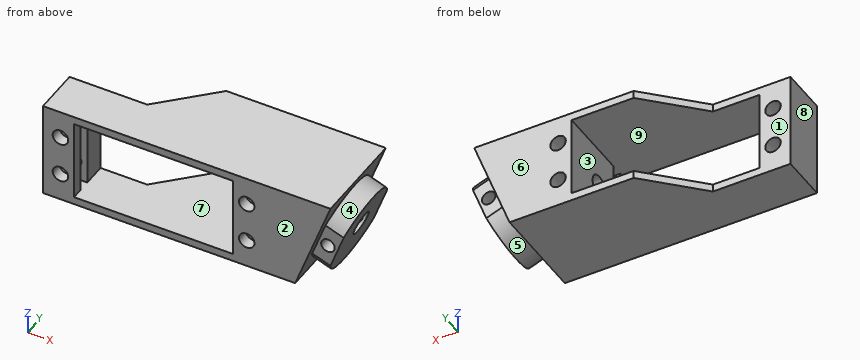
Autodesk Inventor part; units mm, degrees
ref_plane "YZ Plane" through (0, 0, 0) normal (1, 0, 0) x (0, 1, 0)
ref_plane "XZ Plane" through (0, 0, 0) normal (0, 1, 0) x (-1, 0, 0)
ref_plane "XY Plane" through (0, 0, 0) normal (0, 0, 1) x (1, 0, 0)
sketch "Esquisse1" plane through (0, 0, 0) normal (0, 1, 0) x (-1, 0, 0)
  line L0 (20.5, 10.5) -> (-20.5, 10.5)
  line L1 (-20.5, 10.5) -> (-20.5, -10.5)
  line L2 (-20.5, -10.5) -> (20.5, -10.5)
  line L3 (20.5, -10.5) -> (20.5, 10.5)
  line L4 (28.5, 12.5) -> (-36.5, 12.5)
  line L5 (-36.5, 12.5) -> (-36.5, -12.5)
  line L6 (-36.5, -12.5) -> (28.5, -12.5)
  line L7 (28.5, -12.5) -> (28.5, 12.5)
  line L8 (-36.5, -12.5) -> (-45.5993, 12.5)
  line L9 (-45.5993, 12.5) -> (-36.5, 12.5)
  point P0 (0, 0)
  dimension "d0" = 20
  dimension "d1" = 41
  dimension "d2" = 21
  dimension "d3" = 10.5
  dimension "d4" = 20.5
  dimension "d5" = 8
  dimension "d6" = 2
  dimension "d7" = 2
  dimension "d8" = 16
extrude "Extrusion1" add sketch "Esquisse1" along normal mid plane 25
sketch "Esquisse2" plane through (36.5, -12.5, -12.5) normal (0.9397, 0, -0.342) x (-0.342, 0, -0.9397)
  line L0 (-26.6044, 25) -> (0, 0)
  line L1 (0, 0) -> (0, 25)
  line L2 (0, 25) -> (-26.6044, 0)
  arc A0 (-8.3022, 22.298) -> (-18.3022, 22.298) centre (-13.3022, 12.5) ccw
  line L3 (-18.3022, 22.298) -> (-8.3022, 22.298)
  line L4 (-8.3022, 22.298) -> (-8.3022, 2.702)
  line L5 (-8.3022, 2.702) -> (-18.3022, 2.702)
  line L6 (-18.3022, 2.702) -> (-18.3022, 22.298)
  arc A1 (-8.3022, 2.702) -> (-8.3022, 22.298) centre (-13.3022, 12.5) ccw
  arc A2 (-18.3022, 2.702) -> (-8.3022, 2.702) centre (-13.3022, 12.5) ccw
  arc A3 (-18.3022, 22.298) -> (-18.3022, 2.702) centre (-13.3022, 12.5) ccw
  point P0 (0.7376, 12.5)
  dimension "d11" = 22
  dimension "d13" = 10
extrude "Extrusion2" add sketch "Esquisse2" along normal blind 5 contours A3 L6 L0 | L0 L6 L2 A3 | L6 L3 L4 L2 L0 | L0 L2 L6 | L2 L6 A3 | L2 L4 L0 | L0 L4 L5 L6 L2 | A1 L2 L4 | L4 L2 A1 L0 | L0 A1 L4
sketch "Esquisse3" plane through (39.3395, -9.798, -4.6985) normal (0, -1, 0) x (0.9397, 0, -0.342)
  line L0 (5, 10) -> (0, 0)
  line L1 (0, 10) -> (5, 0)
  circle A0 centre (2.5, 5) radius 1.75
  point P0 (-38.574, -9.0398)
  dimension "d16" = 3.5
extrude "Extrusion3" cut sketch "Esquisse3" against normal through all
sketch "Esquisse4" plane through (20.5, -12.5, 10.5) normal (-1, 0, 0) x (0, 0, 1)
  line L0 (-21, 3) -> (0, 3)
  line L1 (0, 3) -> (0, 6)
  line L2 (0, 6) -> (-21, 6)
  line L3 (-21, 6) -> (-21, 3)
  line L4 (-21, 0) -> (-21, 25)
  line L5 (0, 0) -> (0, 25)
  line L6 (0, 0) -> (-21, 0)
  point P0 (-10.5, 12.5)
  dimension "d19" = 3
  dimension "d20" = 3
extrude "Extrusion4" cut sketch "Esquisse4" against normal blind 7 contours L3 L2 L1 L0
sketch "Esquisse5" plane through (-20.5, -12.5, -10.5) normal (1, 0, 0) x (0, 0, -1)
  line L0 (-21, 6) -> (0, 6)
  line L1 (0, 6) -> (0, 3)
  line L2 (0, 3) -> (-21, 3)
  line L3 (-21, 3) -> (-21, 6)
  line L4 (-21, 25) -> (-21, 0)
  line L5 (0, 0) -> (0, 25)
  line L6 (0, 0) -> (-21, 0)
  point P0 (-10.5, 12.5)
  dimension "d23" = 3
  dimension "d24" = 3
extrude "Extrusion5" cut sketch "Esquisse5" against normal blind 7 contours L0 L1 L2 L3
sketch "Esquisse6" plane through (20.5, 12.5, -10.5) normal (-1, 0, 0) x (0, 0, 1)
  line L0 (21, -25) -> (0, 0)
  line L1 (0, -25) -> (21, 0)
  circle A0 centre (10.5, -12.5) radius 3
  dimension "d27" = 6
extrude "Extrusion6" cut sketch "Esquisse6" against normal through all
sketch "Esquisse7" plane through (20.5, 12.5, -10.5) normal (-1, 0, 0) x (0, 0, 1)
  circle A0 centre (10.5, -12.5) radius 3
  circle A1 centre (10.5, -12.5) radius 1.75
  circle A2 centre (10.5, -12.5) radius 3
  dimension "d30" = 0
  dimension "d31" = 3.5
extrude "Extrusion7" add sketch "Esquisse7" against normal blind 18
sketch "Esquisse8" plane through (20.5, 12.5, -10.5) normal (-1, 0, 0) x (0, 0, 1)
  circle A0 centre (10.5, -12.5) radius 3
  dimension "d34" = 6
extrude "Extrusion8" cut sketch "Esquisse8" against normal blind 3
sketch "Esquisse10" plane through (0, -12.5, 0) normal (0, -1, 0) x (1, 0, 0)
  line L0 (-20.5, -10.5) -> (-27.5, -10.5)
  line L1 (-27.5, -10.5) -> (-27.5, 10.5)
  line L2 (-27.5, 10.5) -> (-20.5, 10.5)
  line L3 (-20.5, 10.5) -> (-20.5, -10.5)
  line L4 (20.5, -10.5) -> (27.5, -10.5)
  line L5 (27.5, -10.5) -> (27.5, 10.5)
  line L6 (27.5, 10.5) -> (20.5, 10.5)
  line L7 (20.5, 10.5) -> (20.5, -10.5)
  line L8 (-27.5, -10.5) -> (-27.5, 10.5)
  line L9 (27.5, 10.5) -> (27.5, -10.5)
  line L10 (-27.5, -10.5) -> (-20.5, 0)
  line L11 (-20.5, 0) -> (-27.5, 10.5)
  line L12 (-27.5, 0) -> (-20.5, 10.5)
  line L13 (-20.5, -10.5) -> (-27.5, 0)
  line L14 (20.5, -10.5) -> (27.5, 0)
  line L15 (20.5, 0) -> (27.5, -10.5)
  line L16 (27.5, 10.5) -> (20.5, 0)
  line L17 (20.5, 10.5) -> (27.5, 0)
  circle A0 centre (-24, -5.25) radius 2
  circle A1 centre (24, -5.25) radius 2
  circle A2 centre (24, 5.25) radius 2
  circle A3 centre (-24, 5.25) radius 2
  point P0 (0, 0)
  dimension "d37" = 4
  dimension "d38" = 4
  dimension "d39" = 4
  dimension "d40" = 4
extrude "Extrusion9" cut sketch "Esquisse10" against normal through all contours A0 L10 L13 | L13 L10 A0 | A0 L13 L10 | L10 L13 A0 | A3 L12 L11 | L11 L12 A3 | A3 L11 L12 | L12 L11 A3 | A1 L15 L14 | L14 L15 A1 | L15 L14 A1 | A1 L14 L15 | A2 L17 L16 | L16 L17 A2 | L17 L16 A2 | A2 L16 L17
sketch "Esquisse11" plane through (36.5, 12.5, -12.5) normal (0, 0, -1) x (-1, 0, 0)
  line L0 (65, 0) -> (45, 0)
  line L1 (45, 0) -> (45, -13)
  line L2 (45, -13) -> (65, -13)
  line L3 (65, -13) -> (65, 0)
  line L4 (65, -25) -> (0, -25)
  line L5 (45, -13) -> (32, 0)
  line L6 (0, 0) -> (65, 0)
  line L7 (45, 0) -> (32, 0)
  point P0 (36.5, -12.5)
  dimension "d43" = 20
  dimension "d44" = 12
  dimension "d45" = 45
extrude "Extrusion10" cut sketch "Esquisse11" against normal through all
equation "\"d38\" = d37"
equation "\"d39\" = d37"
equation "\"d40\" = d37"
properties part number "forearm"
Could you check a few things on this model? Use its own coordinates, in mm. Face numbers are marked on the shaded views. A direction names the side the tool comes from. Coordinates: 2 decimals unless noted, no trailing zeros. Order: outer loops, then holes, each group sorted by start corner. A loop starts at its lowest first (then second) coordinate and runs counter-clockwise, first axis right, second up. Notation, with made-up numbers: M -37,70.25 L -29,70.25 A33 cw -29,103.25 Z; hole C 62,-34.5 d5. An arc over 180 degrees is marked long. Use one line per item in the form item = value. Start each with the question number.
1. Suppose I cut it at A-A on x = 0. Write out the boundary of the cut face in (y, z).
2. On a 3-axis mill with a long thin cutter (end or side, diameter ignored), from which of +Z, -Z, +X, -X, +Y, -Y can I reach the whole of each face in a straight line? I mean the marked faces 1, 2, 3, 4 and 5. Say none if no direction works.
3. For pin 1 (6 mm diameter, centred on x = -22.5, z = -1.5, fed in from +Y); pin 2 (5 mm diameter, centred on y = 3, z = 3, fed in from -X); pin 3 (2.5 mm diameter, centred on x = 24, z = 5.25, fed in from +Y); pin 4 (0.9 mm diameter, centred on y = -11.5, z = -1.5, fed in from +X), each with a flat end and sliding along its axis, tell me the tip position at first contact or that it passes through.
4. Suppose I cut it at C-C on z = 0. Count the separate pieces of the cut face and the enclosed holes in it, then the cut area to 3 significant figures.
5. Please list where these lines run through material, in increasing order: line 1 (Z direction, x = -24, y = -3.25); line 2 (X direction, y = -11.05, z = 5.25); line 3 (Y direction, x = 22, z = 7).
6. Suppose I cut it at B-B on x = -24. Write out the boundary of the cut face in (y, z), then the cut area to 3 significant figures.
7. We'd pull the mould along X, two halves only. Please class the marked faces 6, 7, 8 and 9: +X half, -X half, draft (parallel to the pull), parting line (faces both ways), or undercut.
Geometry says:
q1.outline = M -12.5,-12.5 L 8,-12.5 L 8,-10.5 L -12.5,-10.5 Z; M -12.5,10.5 L 8,10.5 L 8,12.5 L -12.5,12.5 Z
q2.face_1 = +Z, -Z, -X, +Y
q2.face_2 = +Z, -Z, +X, -X, -Y
q2.face_3 = +Y, -Y
q2.face_4 = +X
q2.face_5 = -Z
q3.pin_1 = -0.5
q3.pin_2 = 20.5
q3.pin_3 = through
q3.pin_4 = 40.67
q4.separate_pieces = 5
q4.enclosed_holes = 0
q4.area = 513 mm^2
q5.line_1 = -12.5 to -7.25, -3.25 to 3.25, 7.25 to 12.5
q5.line_2 = -28.5 to -26, -22 to -20.5, 20.5 to 22, 26 to 42.96
q5.line_3 = -12.5 to -9.5, -6.5 to 12.5
q6.outline = M -12.5,-12.5 L -0.5,-12.5 L -0.5,-7.25 L -6.5,-7.25 L -6.5,-10.5 L -9.5,-10.5 L -9.5,-7.25 L -12.5,-7.25 Z; M -12.5,-3.25 L -9.5,-3.25 L -9.5,3.25 L -12.5,3.25 Z; M -12.5,7.25 L -9.5,7.25 L -9.5,10.5 L -6.5,10.5 L -6.5,7.25 L -0.5,7.25 L -0.5,12.5 L -12.5,12.5 Z; M -6.5,-3.25 L -0.5,-3.25 L -0.5,3.25 L -6.5,3.25 Z
q6.area = 165 mm^2
q7.face_6 = draft
q7.face_7 = undercut
q7.face_8 = -X half
q7.face_9 = undercut
